The listing builds one solid part. Answer for the finished solid, in the listing's coordinates (mm). Face numbers are marked on the shaded views. A direction names the side the tool comes from. Coordinates: 2 decimals unless noted, no trailing zeros. Order: outer loops, then holes, each group sorted by start corner. A loop starts at its lowest first (then second) coordinate and runs counter-clockwise, first axis right, second up. Notation, with made-up numbers: M 49.25,-29.5 L 101.25,-29.5 A23 ccw 101.25,-2.5 Z; hole C 80,-2 d1. An arc over 180 degrees is marked long. One line per item, written item: value. Start each with the question number.
Q1. This flat-tipped pin is pushed along its axis until it touches: pin 1 Ø0.7 at (x, y) = (42, 6) entering from +Z. Where does it stop, or does it pass through?
Q2. For the marked faces 5, 6 and 7, determine the directions among +Z, -Z, +X, -X, +Y, -Y from which every point of the face is accessible in a straight line to the end or side of a thin tool.
Q3. The part is cut by section A-A on x = 13. Give the vertices of the cut face in (y, z).
Q4. The part is cut by section B-B on z = 14. Give the number of separate pieces and of enclosed holes in the cut face, then the cut area to 3 significant figures.
Q5. Determine the mould class of the marked faces 1, 2, 3 and 4 for opening direction Y: pulls with the +Y half, pulls with the -Y half, needs draft (parallel to the pull), parting line crosses it, or undercut.
Q6. The part is cut by section D-D on x = 25. Give the vertices of the cut face in (y, z).
Q7. Straight lines are drawn through the part: line 1 along Y through (x, z) = (21, 9.25); line 2 along X through (y, z) = (5.25, 8.5); line 3 along Y through (x, z) = (25, 10). For each, find the intervals that lie inside material, in ascending order. Write a range as [from, to].
```python
from build123d import *

# Parameters (mm, degrees)
SKETCH_1_W          = 50
SKETCH_1_H          = 10.5
EXTRUDE_1_DEPTH     = 17
SKETCH_2_W          = 36
SKETCH_2_H          = 3.5
CUT_EXTRUDE_1_DEPTH = 10
CUT_EXTRUDE_2_DEPTH = 10.5
SKETCH_4_W          = 3.5
SKETCH_4_H          = 6.5
CUT_EXTRUDE_3_DEPTH = 6.5
FILLET_1_R          = 2
SKETCH_6_R          = 3
SKETCH_6_R_2        = 1.75
CUT_EXTRUDE_4_DEPTH = 18
CUT_EXTRUDE_5_DEPTH = 11
CUT_EXTRUDE_6_DEPTH = 3
SKETCH_9_W          = 58.421136066
SKETCH_9_H          = 24.245128271
CUT_EXTRUDE_7_DEPTH = 7.5


with BuildPart() as part:
    # ｽｹｯﾁ1 → ﾎﾞｽ - 押し出し1 (new body)
    with BuildSketch(Plane.XY):
        with Locations((25, 5.25)):
            Rectangle(SKETCH_1_W, SKETCH_1_H)
    extrude(amount=EXTRUDE_1_DEPTH)

    # ｽｹｯﾁ2 → ｶｯﾄ - 押し出し1 (cut)
    with BuildSketch(Plane.XY.offset(17)):
        with Locations((25, 5.25)):
            Rectangle(SKETCH_2_W, SKETCH_2_H)
    extrude(amount=-CUT_EXTRUDE_1_DEPTH, mode=Mode.SUBTRACT)

    # ｽｹｯﾁ3 → ｶｯﾄ - 押し出し2 (cut)
    with BuildSketch(Plane.XZ):
        Polygon((1, 17), (3, 12), (7, 12), (17, 17), align=None)
        Polygon((33, 17), (43, 12), (47, 12), (49, 17), align=None)
    extrude(amount=-CUT_EXTRUDE_2_DEPTH, mode=Mode.SUBTRACT)

    # ｽｹｯﾁ4 → ｶｯﾄ - 押し出し3 (cut)
    with BuildSketch(Plane(origin=(0, 0, 0), x_dir=(-1, 0, 0), z_dir=(0, 0, -1))):
        with Locations((-2.15, 5.25)):
            Rectangle(SKETCH_4_W, SKETCH_4_H)
        with Locations((-47.85, 5.25)):
            Rectangle(SKETCH_4_W, SKETCH_4_H)
    extrude(amount=-CUT_EXTRUDE_3_DEPTH, mode=Mode.SUBTRACT)

    # ﾌｨﾚｯﾄ1
    fillet_1_edges = [part.edges().sort_by_distance(p)[0] for p in [
        (0, 0, 8.5),
        (0, 10.5, 8.5),
        (50, 0, 8.5),
        (50, 10.5, 8.5),
    ]]
    fillet(fillet_1_edges, radius=FILLET_1_R)

    # ｽｹｯﾁ6 → ｶｯﾄ - 押し出し4 (cut, through all)
    with BuildSketch(Plane(origin=(0, 0, 0), x_dir=(-1, 0, 0), z_dir=(0, 0, -1))):
        with Locations((-25, 5.25)):
            Circle(SKETCH_6_R)
        with Locations((-11.75, 5.25)):
            Circle(SKETCH_6_R_2)
        with Locations((-38.25, 5.25)):
            Circle(SKETCH_6_R_2)
    extrude(amount=-CUT_EXTRUDE_4_DEPTH, mode=Mode.SUBTRACT)

    # ｽｹｯﾁ7 → ｶｯﾄ - 押し出し5 (cut, through all)
    with BuildSketch(Plane.XY.offset(7)):
        Polygon((34.785898385, 5.25), (36.517949192, 2.25), (39.982050808, 2.25), (41.714101615, 5.25), (39.982050808, 8.25), (36.517949192, 8.25), align=None)
        Polygon((13.482050808, 8.25), (15.214101615, 5.25), (13.482050808, 2.25), (10.017949192, 2.25), (8.285898385, 5.25), (10.017949192, 8.25), align=None)
    extrude(amount=CUT_EXTRUDE_5_DEPTH, mode=Mode.SUBTRACT)

    # ｽｹｯﾁ8 → ｶｯﾄ - 押し出し6 (cut)
    with BuildSketch(Plane.XY.offset(7)):
        Polygon((36.517949192, 2.25), (39.982050808, 2.25), (41.714101615, 5.25), (39.982050808, 8.25), (36.517949192, 8.25), (34.785898385, 5.25), align=None)
        Polygon((15.214101615, 5.25), (13.482050808, 2.25), (10.017949192, 2.25), (8.285898385, 5.25), (10.017949192, 8.25), (13.482050808, 8.25), align=None)
    extrude(amount=-CUT_EXTRUDE_6_DEPTH, mode=Mode.SUBTRACT)

    # ｽｹｯﾁ9 → ｶｯﾄ - 押し出し7 (cut, through all)
    with BuildSketch(Plane(origin=(0, 0, 6.5), x_dir=(-1, 0, 0), z_dir=(0, 0, -1))):
        with Locations((-24.970881096, 5.810967265)):
            Rectangle(SKETCH_9_W, SKETCH_9_H)
    extrude(amount=CUT_EXTRUDE_7_DEPTH, mode=Mode.SUBTRACT)


solid = part.part
```
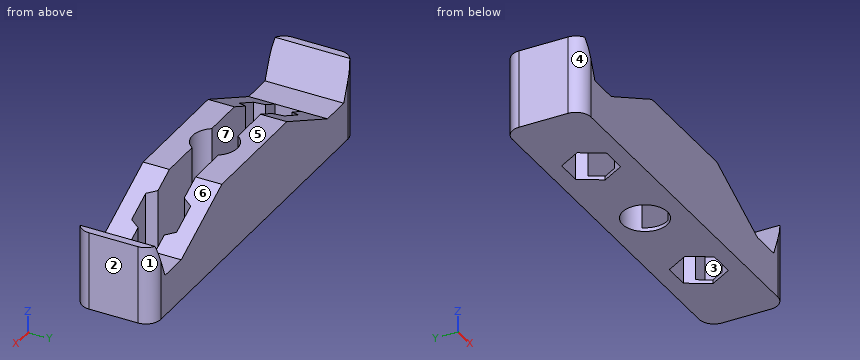
Output:
1. pin 1: stops at z = 7
2. face 5: +Z, +X, -X, +Y, -Y
2. face 6: +Z, +Y, -Y
2. face 7: +Z
3. outline: M 0,6.5 L 2.25,6.5 L 2.25,15 L 0,15 Z; M 8.25,6.5 L 10.5,6.5 L 10.5,15 L 8.25,15 Z
4. separate pieces: 4
4. enclosed holes: 0
4. area: 216 mm^2
5. face 1: pulls with the +Y half
5. face 2: needs draft
5. face 3: undercut
5. face 4: pulls with the -Y half
6. outline: M 0,6.5 L 2.25,6.5 L 2.25,17 L 0,17 Z; M 8.25,6.5 L 10.5,6.5 L 10.5,17 L 8.25,17 Z
7. line 1: y = [0, 3.5], [7, 10.5]
7. line 2: x = [0, 7], [43, 50]
7. line 3: y = [0, 2.25], [8.25, 10.5]
